Here's how the part is built. I have some questions about the finished solid (model axes, mm). A direction names the side the tool comes from. Coordinates: 2 decimals unless noted, no trailing zeros. Write each loop counter-clockwise with the first axis right and the second up, starting at its lowest first coordinate (ties: lowest second). Pieces come first, ordered by that corner, then holes. Notation, with made-up numbers: (85.25, 6.5) - (141.25, 6.5) arc R12 cw to (141.25, 13.5) - close; hole circle Ø3 at (13.5, -12). An arc over 180 degrees is marked (long way). Answer in a Markdown table with one row per item. Add a question column.
Item 1: We'd pull the mould along X, two halves only. Please class faces 1 (the face through (0.45, 4.47, 1.43)), 2 (the face through (-2, 2.5, 0)), 3 (the face through (0.203, 4.472, 0.644)): +X half, -X half, draft (parallel to the pull), parting line (faces both ways), or undercut.
Item 2: Imagine slicing it at C-C (x = 3.5). Please give me the cut outline in (y, z).
Item 3: I'm going to push flat-ended pins straight in: pin 1 (5 mm diameter, centred on x = 1.5, z = 2.5, fed in from +Y); pin 2 (2 mm diameter, centred on x = -3, y = 1.5, fed in from -Z); pin 3 (1 mm diameter, centred on x = -3.5, y = 3.5, fed in from +Z). Where does each tip first touch, or does it pass through?
Item 4: Which directions (+Z, -Z, +X, -X, +Y, -Y) give clear straight access to the entire face, cutting with the end or side of a thin tool? Please do faces 4 (the face through (0, 0, 0)), 5 (the face through (-0.397, 1.514, -0.088)).
Item 5: If I drill on probe 1 along X at (y, z) = (1.8, 0); probe 2 along Y at (x, z) = (3.25, 0); probe 3 along Y at (x, z) = (2.5, -2), over which ranges is the centre line in solid material (lowest first)? Write a range as from..to.
Item 6: Imagine slicing it at D-D (z = 1.25). Please give me the cut outline in (x, y), plus the area to 3 significant figures.
from build123d import *

# Parameters (mm, degrees)
SKETCH1_R           = 4.5
BOSS_EXTRUDE1_DEPTH = 2.5
SKETCH2_R           = 1.5
SKETCH2_R_2         = 0.675
BOSS_EXTRUDE2_DEPTH = 4
SKETCH3_W           = 4.5
SKETCH3_H           = 0.25
SKETCH5_R           = 0.406492391
CUT_EXTRUDE2_DEPTH  = 2


with BuildPart() as part:
    # Sketch1 → Boss-Extrude1 (new body)
    with BuildSketch(Plane(origin=(0, 0, 0), x_dir=(1, 0, 0), z_dir=(0, 1, 0))):
        with Locations(Location((0, 0, 0), (0, 0, 270))):
            Circle(SKETCH1_R)
    extrude(amount=BOSS_EXTRUDE1_DEPTH)

    # Sketch2 → Boss-Extrude2 (add)
    with BuildSketch(Plane(origin=(0, 2.5, 0), x_dir=(1, 0, 0), z_dir=(0, 1, 0))):
        with Locations(Location((0, 0, 0), (0, 0, 270))):
            Circle(SKETCH2_R)
        with Locations(Location((0, 0, 0), (0, 0, 270))):
            Circle(SKETCH2_R_2, mode=Mode.SUBTRACT)
    extrude(amount=BOSS_EXTRUDE2_DEPTH)

    # Sketch3 → Cut-Revolve1 (revolve, cut)
    with BuildSketch(Plane.XY, mode=Mode.PRIVATE) as cut_revolve1_sk:
        with Locations((2.25, 1.375)):
            Rectangle(SKETCH3_W, SKETCH3_H)
    revolve(cut_revolve1_sk.sketch.rotate(Axis((0, 1.25, 0), (1, 0, 0)), 90), axis=Axis((0, 1.25, 0), (1, 0, 0)), mode=Mode.SUBTRACT)

    # Sketch5 → Cut-Extrude2 (cut)
    with BuildSketch(Plane(origin=(0, 2.5, 0), x_dir=(1, 0, 0), z_dir=(0, 1, 0))):
        with Locations(Location((0, 0, 0), (0, 0, 270))):
            Circle(SKETCH5_R)
    extrude(amount=-CUT_EXTRUDE2_DEPTH, mode=Mode.SUBTRACT)


solid = part.part
Here are the results:
| question | item | result |
|---|---|---|
| 1 | face 1 | parting line |
| 1 | face 2 | draft |
| 1 | face 3 | undercut |
| 2 | outline | (0, -2.83) - (2.5, -2.83) - (2.5, 2.83) - (0, 2.83) - close; hole circle Ø0.5 at (1.25, 0) |
| 3 | pin 1 | stops at y = 6.5 |
| 3 | pin 2 | stops at z = -4.03 |
| 3 | pin 3 | passes through |
| 4 | face 4 | +Z, -Z, +X, -X, -Y |
| 4 | face 5 | +Y |
| 5 | probe 1 | x = -4.5..-0.41, 0.41..4.5 |
| 5 | probe 2 | y = 0..1, 1.5..2.5 |
| 5 | probe 3 | y = 0..2.5 |
| 6 | outline | (-4.32, 0) - (4.32, 0) - (4.32, 2.5) - (0.83, 2.5) - (0.83, 6.5) - (-0.83, 6.5) - (-0.83, 2.5) - (-4.32, 2.5) - close |
| 6 | area | 28.2 mm2 |
